```python
from build123d import *

# Parameters (mm, degrees)
SKETCH1_R               = 22.5
BOSS_EXTRUDE1_DEPTH     = 30
SKETCH2_R               = 17.5
CUT_EXTRUDE1_DEPTH      = 15
F_1_4_20_TAPPED_HOLE1_D = 5.1054
CHAMFER1_SIZE           = 12.7


with BuildPart() as part:
    # Sketch1 → Boss-Extrude1 (new body)
    with BuildSketch(Plane.XY):
        Circle(SKETCH1_R)
    extrude(amount=-BOSS_EXTRUDE1_DEPTH)

    # Sketch2 → Cut-Extrude1 (cut)
    with BuildSketch(Plane(origin=(0, 0, -30), x_dir=(-1, 0, 0), z_dir=(0, 0, -1))):
        Circle(SKETCH2_R)
    extrude(amount=-CUT_EXTRUDE1_DEPTH, mode=Mode.SUBTRACT)

    # 1/4-20 Tapped Hole1 (through all)
    with Locations(Plane.XY):
        with Locations((0, 0)):
            Hole(F_1_4_20_TAPPED_HOLE1_D / 2)

    # Chamfer1
    chamfer1_edges = [part.edges().sort_by_distance(p)[0] for p in [
        (-22.5, 0, 0),
    ]]
    chamfer(chamfer1_edges, length=CHAMFER1_SIZE)


solid = part.part
```
Design review of the part built by this model. Coordinates are the model's own, in mm. A direction names the side the tool comes from. Give positions to 0.01 mm unless a question says otherwise; leave off trailing zeros. Loops run counter-clockwise (first coordinate to the right, second up) from the corner with the lowest first, then second, coordinate; pieces in that order, holes last. Notation, with made-up numbers: (-15.5, -31) -> (-10.5, -31) arc R11 cw to (-10.5, -19) -> close; hole circle Ø9 at (39.25, 13.5). An arc over 180 degrees is marked (long way). One line per item, written item: value.
Q1. We need section A-A on y = 0. Give the boundary of the cut face in (x, z).
Numbers:
outline: (-22.5, -30) -> (-17.5, -30) -> (-17.5, -15) -> (-2.55, -15) -> (-2.55, 0) -> (-9.8, 0) -> (-22.5, -12.7) -> close; (2.55, -15) -> (17.5, -15) -> (17.5, -30) -> (22.5, -30) -> (22.5, -12.7) -> (9.8, 0) -> (2.55, 0) -> close
Q2. We need section D-D on z = -17. Give the boundary of the cut face in (x, y).
Numbers:
outline: circle Ø45 at (0, 0); hole circle Ø35 at (0, 0)
Q3. Machinability: for faces 1 (the cylindrical face through (10.382, -19.961, -21.229)), 2 (the flat face through (0, -4, -15)), which of the approach directions +Z, -Z, +X, -X, +Y, -Y give a long, thin tool a straight path to every point of the face, cutting with its end or side? Answer none if there is none.
Numbers:
face 1: +Z, -Z
face 2: -Z
Q4. Draft analysis for pull direction Y (two halves, no side actions). For faces 3 (the flat face through (12, -13, -30)), 4 (the cylindrical face through (-2.435, 0.767, -7.605)), 5 (the conical face through (-8.27, -6.34, -0.62)), state which applies: pulls with the +Y half, pulls with the -Y half, needs draft (parallel to the pull), parting line crosses it, or undercut.
Numbers:
face 3: needs draft
face 4: undercut
face 5: parting line crosses it
Q5. For L1, parallel to Z at x = 6.5, y = -1.5; L2, parallel to X at y = 8, z = -21; L3, parallel to Y at x = 0, z = -20.5, list the stretches that pass through material, from the lowest coordinate up.
Numbers:
L1: z = -15 to 0
L2: x = -21.03 to -15.56, 15.56 to 21.03
L3: y = -22.5 to -17.5, 17.5 to 22.5
Q6. For pin 1 Ø10 at (x, y) = (-0.5, 11.5) entering from +Z; pin 2 Ø6 at (x, z) = (8, -13) entering from -Y; pin 3 Ø4 at (x, y) = (1, -15) entering from +Z; pin 4 Ø5 at (y, z) = (-17.5, -18.5) entering from +X, all flat-tipped, find the tip position at first contact; note any pin that passes through.
Numbers:
pin 1: stops at z = 0
pin 2: stops at y = -21.94
pin 3: stops at z = -3.23
pin 4: stops at x = 16.77
Q7. We need section C-C on z = -7.5. Give the boundary of the cut face in (x, y).
Numbers:
outline: circle Ø34.6 at (0, 0); hole circle Ø5.11 at (0, 0)
